Verification items for the finished model (mm, model axes). A direction names the side the tool comes from. Give positions to 0.01 mm unless a question says otherwise; leave off trailing zeros. Order: outer loops, then holes, each group sorted by start corner. A loop starts at its lowest first (then second) coordinate and runs counter-clockwise, first axis right, second up. Notation, with made-up numbers: (61.25, -11.75) - (90.25, -11.75) arc R17 cw to (90.25, 12.25) - close; hole circle Ø1 at (11.5, 39.25). An arc over 180 degrees is marked (long way). Answer as a JSON object with one key per item and string values.
```python
from build123d import *

# Parameters (mm, degrees)
SKETCH1_R           = 105.177936238
SKETCH1_R_2         = 79.476526286
BOSS_EXTRUDE1_DEPTH = 5
SKETCH3_W           = 25.87147266
SKETCH3_H           = 5
CUT_EXTRUDE1_DEPTH  = 5
CIRPATTERN1_COUNT   = 9
CIRPATTERN1_ANGLE   = 240


with BuildPart() as part:
    # Sketch1 → Boss-Extrude1 (new body)
    with BuildSketch(Plane(origin=(0, 0, 0), x_dir=(1, 0, 0), z_dir=(0, 1, 0))):
        Circle(SKETCH1_R)
        Circle(SKETCH1_R_2, mode=Mode.SUBTRACT)
    extrude(amount=BOSS_EXTRUDE1_DEPTH)

    # Sketch2 → Cut-Revolve1 (revolve, cut)
    with BuildSketch(Plane.XY):
        Polygon((105.177936238, 0), (105.037977295, 6.300404607), (110.743312601, 6.300404607), (110.743312601, 0), align=None)
    revolve(axis=Axis((0, 0, 0), (0, 1, 0)), mode=Mode.SUBTRACT)

    # Sketch3 → Cut-Extrude1 (cut)
    with BuildSketch(Plane(origin=(0, 5, 0), x_dir=(1, 0, 0), z_dir=(0, 1, 0))):
        with Locations((76.959203751, 0)):
            Rectangle(SKETCH3_W, SKETCH3_H)
    cut_extrude1 = extrude(amount=-CUT_EXTRUDE1_DEPTH, mode=Mode.SUBTRACT)

    # CirPattern1: Cut-Extrude1 ×9 about axis
    cirpattern1_axis = Axis((0, 0, 0), (0, -1, 0))
    for i in range(1, CIRPATTERN1_COUNT):
        add(cut_extrude1.rotate(cirpattern1_axis, i * CIRPATTERN1_ANGLE / (CIRPATTERN1_COUNT - 1)), mode=Mode.SUBTRACT)


solid = part.part
```
(1) Section check B-B (z = 0). Record the cut outline in (x, y), then the cut area to 3 significant figures.
Computed values:
{"outline": "(-105.18, 0) - (-89.89, 0) - (-89.89, 5) - (-105.07, 5) - close; (89.89, 0) - (105.18, 0) - (105.07, 5) - (89.89, 5) - close", "area": "152 mm²"}
(2) Material ranges on line 1 along X through (y, z) = (0.5, 42.5); line 2 along Z through (x, y) = (-73, 1.75); line 3 along X through (y, z) = (3.8, 43), recorded low to high. Write a range as [from, to].
Computed values:
{"line 1": "x = [-96.2, -78.61], [-68.61, -67.16], [67.16, 68.61], [78.61, 96.2]", "line 2": "z = [-75.67, -45.03], [-39.26, -31.42], [31.42, 39.26], [45.03, 75.67]", "line 3": "x = [-95.89, -78.98], [-69.48, -66.84], [66.84, 69.48], [78.98, 95.89]"}
(3) Gauge pin test, flat ends, axial feed: pin 1 Ø2 at (y, z) = (0.5, 18) entering from -X; pin 2 Ø1.5 at (y, z) = (2.5, 73) entering from -X; pin 3 Ø1.5 at (x, y) = (84, 2.5) entering from -Z. Record the tip position at first contact, or that the pin passes through.
Computed values:
{"pin 1": "stops at x = -103.79", "pin 2": "stops at x = -76.36", "pin 3": "stops at z = -64.19"}
(4) Access from +Z, -Z, +X, -X, +Y, -Y to the whole of each face (thin tool, end or side, straight path). Record for faces 4 (the flat face through (23, 5, 77)), 5 (the cylindrical face through (20.322, 2.465, 76.834)).
Computed values:
{"face 4": "+Z, -Z, +X, -X, +Y", "face 5": "+Y, -Y"}
(5) Release check for a two-part mould opening along X. For faces 1 (the conical face through (100.22, 4.76, -31.56)), 2 (the flat face through (-74.51, 2.54, 40.13)), 3 (the flat face through (23, 0, 77)) record: pulls with the +X half, pulls with the -X half, needs draft (parallel to the pull), parting line crosses it, or undercut.
Computed values:
{"face 1": "parting line crosses it", "face 2": "undercut", "face 3": "needs draft"}
(6) Section check A-A (x = 0). Record the cut outline in (y, z).
Computed values:
{"outline": "(0, -105.18) - (5, -105.07) - (5, -79.48) - (0, -79.48) - close; (0, 89.89) - (5, 89.89) - (5, 105.07) - (0, 105.18) - close"}
